Design review of the part built by this model. Coordinates are the model's own, in mm. A direction names the side the tool comes from. Coordinates: 2 decimals unless noted, no trailing zeros. Loops run counter-clockwise (first coordinate to the right, second up) from the corner with the lowest first, then second, coordinate; pieces in that order, holes last.
Q1. For P1, Ø4, axis at x = 311.5, y = -13.5, coming from the +Z side; P2, Ø8, axis at x = 305, z = -25.5, coming from the -Y side; P3, Ø5, axis at x = 309, z = -25, coming from the -Y side, all flat-tipped, find the tip position at first contact; note any pin that passes through.
Q2. Draft analysis for pull direction X (two halves, no side actions). For faces 1 (the face through (327, -13, -40)), 2 (the face through (333.14, 5.15, -27.45)), 3 (the face through (332.27, 5, -11.09)), state which applies: released by +X, released by -X, zero draft, split by the parting line, or undercut.
Q3. Add section A-A on y = 7.5. Give the boundary of the cut face in (x, z), and give its area (3 significant figures).
Q4. Wall thickness on probe 1 along X at (y, z) = (0, -34); probe 2 along Y at (x, z) = (303.5, -31); probe 3 along X at (y, z) = (0, -16): over which ranges is each line inside the solid? List them lowest first.
Q5. Add section B-B on z = -18. Give the boundary of the cut face in (x, y).
Q6. Add section C-C on z = -25. Give the boundary of the cut face in (x, y).
Q7. Machinability: for faces 4 (the face through (300.399, -0.06, -16.736)), 5 (the face through (332.187, 4.851, -28.164)), which of the approach directions +Z, -Z, +X, -X, +Y, -Y give a long, thin tool a straight path to every point of the face, cutting with its end or side? Answer none if there is none.
```python
from build123d import *

# Parameters (mm, degrees)
SKETCH1_R           = 17.15
SKETCH1_R_2         = 16.15
BOSS_EXTRUDE1_DEPTH = 40
SKETCH2_R           = 22.225
CUT_EXTRUDE1_DEPTH  = 352.453482
SKETCH3_R           = 19.05
CUT_EXTRUDE2_DEPTH  = 52.6500001


with BuildPart() as part:
    # Sketch1 → Boss-Extrude1 (new body)
    with BuildSketch(Plane.XY):
        with Locations((316.783091477, 0)):
            Circle(SKETCH1_R)
        with Locations((316.783091477, 0)):
            Circle(SKETCH1_R_2, mode=Mode.SUBTRACT)
    extrude(amount=-BOSS_EXTRUDE1_DEPTH)

    # Sketch2 → Cut-Extrude1 (cut)
    with BuildSketch(Plane(origin=(-60.87597301, 0, 29.691195898), x_dir=(-0.438371147, 0, -0.898794046), z_dir=(0.898794046, 0, -0.438371147))):
        with Locations((-138.868567094, 0)):
            Circle(SKETCH2_R)
    extrude(amount=CUT_EXTRUDE1_DEPTH, mode=Mode.SUBTRACT)

    # Sketch3 → Cut-Extrude2 (cut, through all)
    with BuildSketch(Plane.XZ.offset(34.5)):
        with Locations((316.783091477, 0)):
            Circle(SKETCH3_R)
    extrude(amount=-CUT_EXTRUDE2_DEPTH, mode=Mode.SUBTRACT)


solid = part.part
```
Entries:
1. P1: stops at z = -17.73
1. P2: stops at y = -15.28
1. P3: stops at y = -16.32
2. face 1: zero draft
2. face 2: split by the parting line
2. face 3: undercut
3. outline: (301.36, -40) - (302.48, -40) - (302.48, -16.3) - (301.36, -15.75) - close; (331.09, -40) - (332.21, -40) - (332.21, -11.18) arc R19.05 cw to (331.09, -12.58) - close
3. area: 58.3 mm2
4. probe 1: x = 299.63 to 300.63, 332.93 to 333.93
4. probe 2: y = -10.85 to -9.19, 9.19 to 10.85
4. probe 3: x = 332.93 to 333.93
5. outline: (310.55, -15.98) - (310.55, -14.9) arc R16.15 cw to (310.55, 14.9) - (310.55, 15.98) arc R17.15 ccw to start; (323.02, -15.98) arc R17.15 ccw to (323.02, 15.98) - (323.02, 14.9) arc R16.15 cw to (323.02, -14.9) - close
6. outline: circle Ø34.3 at (316.78, 0); hole circle Ø32.3 at (316.78, 0)
7. face 4: +Z
7. face 5: +Z, -Z
